Geometry check sheet. Reference: the model listing, model coordinates, mm. A direction names the side the tool comes from. Round coordinates to 2 decimals unless told otherwise and drop trailing zeros. Write each loop counter-clockwise with the first axis right and the second up, starting at its lowest first coordinate (ties: lowest second). Pieces come first, ordered by that corner, then holes. Notation, with made-up numbers: (46.5, -12.75) -> (82.5, -12.75) arc R17 ccw to (82.5, 0.25) -> close; hole circle Ø1 at (20, 69). An arc over 180 degrees is marked (long way). Return JSON: item names as keys, results as strings. Group by question number.
from build123d import *

# Parameters (mm, degrees)
F0_R     = 63.5
F0_R_2   = 62.2
F1_DEPTH = 22
F2_R     = 63.5
F2_R_2   = 56.5
F3_DEPTH = 2
F4_SIZE  = 1


with BuildPart() as f1:
    # F0 (on Top) → F1 (new body)
    with BuildSketch(Plane.XY):
        Circle(F0_R)
        Circle(F0_R_2, mode=Mode.SUBTRACT)
    extrude(amount=F1_DEPTH)

    # F2 (on Top) → F3 (join)
    with BuildSketch(Plane.XY):
        Circle(F2_R)
        Circle(F2_R_2, mode=Mode.SUBTRACT)
    extrude(amount=-F3_DEPTH)

    # F4
    f4_edges = [f1.edges().sort_by_distance(p)[0] for p in [
        (-63.5, 0, -2),
    ]]
    chamfer(f4_edges, length=F4_SIZE)


solid = f1.part
1) Material ranges on probe 1 along Y at (x, z) = (0, -0.8); probe 2 along X at (y, z) = (1.5, 6.5); probe 3 along Y at (x, z) = (0, 11.75), recorded low to high. Write a range as [from, to].
2) Tool access check on faces 1 (the face through (-47, -32, -2)), 2 (the face through (-13.48, -60.72, 10.85)). Record the directions out of +Z, -Z, +X, -X, +Y, -Y that give a thin tool (end or side, any length) a straight path to the whole face; none if there is none.
3) Sectioned sample at C-C on z = 11.5. Enter the section's corners in (x, y).
4) Mould release check, pull along X, two halves, no side actions. Record for faces 3 (the face through (14, -55, 0)), 4 (the face through (42, -47, 22)), 5 (the face through (-13.77, -61.99, 10.66)), 6 (the face through (30.374, 47.641, -0.986)): +X half, -X half, draft (parallel to the pull), parting line (faces both ways), or undercut.
5) Go/stop test with flat-tipped pins: P1, Ø1.5, axis at x = -22.5, z = 5, coming from the -Y side; P2, Ø3, axis at x = 9.5, z = 11, coming from the +Y side; P3, Ø1, axis at x = -39, z = 3.5, coming from the +Y side. Record where each tip stops, or that it passes through.
6) Sectioned sample at A-A on y = 0. Enter the section's corners in (x, z), and give its area (3 significant figures).
Evaluation:
{
 "1": {"probe 1": "y = [-63.5, -56.5], [56.5, 63.5]", "probe 2": "x = [-63.48, -62.18], [62.18, 63.48]", "probe 3": "y = [-63.5, -62.2], [62.2, 63.5]"},
 "2": {"face 1": "-Z, +X, -X, +Y, -Y", "face 2": "+Z"},
 "3": {"outline": "circle Ø127 at (0, 0); hole circle Ø124.4 at (0, 0)"},
 "4": {"face 3": "undercut", "face 4": "draft", "face 5": "parting line", "face 6": "undercut"},
 "5": {"P1": "stops at y = -59.66", "P2": "stops at y = 62.99", "P3": "stops at y = 50.5"},
 "6": {"outline": "(-63.5, -1) -> (-62.5, -2) -> (-56.5, -2) -> (-56.5, 0) -> (-62.2, 0) -> (-62.2, 22) -> (-63.5, 22) -> close; (56.5, -2) -> (62.5, -2) -> (63.5, -1) -> (63.5, 22) -> (62.2, 22) -> (62.2, 0) -> (56.5, 0) -> close", "area": "84.2 mm2"}
}
